Here's how the part is built. I have some questions about the finished solid (model axes, mm). A direction names the side the tool comes from. Round coordinates to 2 decimals unless told otherwise and drop trailing zeros. Loops run counter-clockwise (first coordinate to the right, second up) from the corner with the lowest first, then second, coordinate; pieces in that order, holes last. Notation, with made-up numbers: M 64,41 L 108,41 A9 ccw 108,55 Z; hole C -8,-18 d11. An arc over 180 degrees is marked long. Answer as a JSON object with one key per item and string values.
from build123d import *

# Parameters (mm, degrees)
F0_R     = 3.302
F1_DEPTH = 12.7


with BuildPart() as f1:
    # F0 (on Top) → F1 (new body)
    with BuildSketch(Plane.XY):
        with BuildLine():
            ThreePointArc((24.764251, -5.647288), (25.240562, -2.84148), (25.4, 0))
            ThreePointArc((25.4, 0), (25.399308, 0.187557), (25.39723, 0.375103))
            ThreePointArc((25.39723, 0.375103), (25.260856, 2.655023), (24.920228, 4.913475))
            ThreePointArc((24.920228, 4.913475), (24.156836, 7.849032), (23.048956, 10.672658))
            ThreePointArc((23.048956, 10.672658), (21.997045, 12.7), (20.767271, 14.624652))
            ThreePointArc((20.767271, 14.624652), (18.875879, 16.995917), (16.715308, 19.124813))
            ThreePointArc((16.715308, 19.124813), (14.929745, 20.549032), (13.023464, 21.807095))
            ThreePointArc((13.023464, 21.807095), (10.331111, 23.204055), (7.491431, 24.270115))
            ThreePointArc((7.491431, 24.270115), (5.280957, 24.844949), (3.027782, 25.218892))
            ThreePointArc((3.027782, 25.218892), (0, 25.4), (-3.027782, 25.218892))
            ThreePointArc((-3.027782, 25.218892), (-5.280957, 24.844949), (-7.491431, 24.270115))
            ThreePointArc((-7.491431, 24.270115), (-10.331111, 23.204055), (-13.023464, 21.807095))
            ThreePointArc((-13.023464, 21.807095), (-14.929745, 20.549032), (-16.715308, 19.124813))
            ThreePointArc((-16.715308, 19.124813), (-18.875879, 16.995917), (-20.767271, 14.624652))
            ThreePointArc((-20.767271, 14.624652), (-21.997045, 12.7), (-23.048956, 10.672658))
            ThreePointArc((-23.048956, 10.672658), (-24.156836, 7.849032), (-24.920228, 4.913475))
            ThreePointArc((-24.920228, 4.913475), (-25.260856, 2.655023), (-25.39723, 0.375103))
            ThreePointArc((-25.39723, 0.375103), (-25.260856, -2.655023), (-24.764251, -5.647288))
            ThreePointArc((-24.764251, -5.647288), (-24.156836, -7.849032), (-23.354093, -9.98731))
            ThreePointArc((-23.354093, -9.98731), (-21.997045, -12.7), (-20.326311, -15.231582))
            ThreePointArc((-20.326311, -15.231582), (-18.875879, -16.995917), (-17.27282, -18.622827))
            ThreePointArc((-17.27282, -18.622827), (-14.929745, -20.549032), (-12.373766, -22.182198))
            ThreePointArc((-12.373766, -22.182198), (-10.331111, -23.204055), (-8.20492, -24.038288))
            ThreePointArc((-8.20492, -24.038288), (-5.280957, -24.844949), (-2.281685, -25.29731))
            ThreePointArc((-2.281685, -25.29731), (0, -25.4), (2.281685, -25.29731))
            ThreePointArc((2.281685, -25.29731), (5.280957, -24.844949), (8.20492, -24.038288))
            ThreePointArc((8.20492, -24.038288), (10.331111, -23.204055), (12.373766, -22.182198))
            ThreePointArc((12.373766, -22.182198), (14.929745, -20.549032), (17.27282, -18.622827))
            ThreePointArc((17.27282, -18.622827), (18.875879, -16.995917), (20.326311, -15.231582))
            ThreePointArc((20.326311, -15.231582), (21.997045, -12.7), (23.354093, -9.98731))
            ThreePointArc((23.354093, -9.98731), (24.156836, -7.849032), (24.764251, -5.647288))
        make_face()
        Circle(F0_R, mode=Mode.SUBTRACT)
        with BuildLine():
            ThreePointArc((25.39723, 0.375103), (25.399308, 0.187557), (25.4, 0))
            ThreePointArc((25.4, 0), (25.240562, -2.84148), (24.764251, -5.647288))
            Line((24.764251, -5.647288), (30.631833, -3.219535))
            Line((30.631833, -3.219535), (25.39723, 0.375103))
        make_face()
        with BuildLine():
            ThreePointArc((23.048956, 10.672658), (24.156836, 7.849032), (24.920228, 4.913475))
            Line((24.920228, 4.913475), (29.293075, 9.517897))
            Line((29.293075, 9.517897), (23.048956, 10.672658))
        make_face()
        with BuildLine():
            Line((26.674069, -15.400281), (23.354093, -9.98731))
            ThreePointArc((23.354093, -9.98731), (21.997045, -12.7), (20.326311, -15.231582))
            Line((20.326311, -15.231582), (26.674069, -15.400281))
        make_face()
        with BuildLine():
            ThreePointArc((16.715308, 19.124813), (18.875879, 16.995917), (20.767271, 14.624652))
            Line((20.767271, 14.624652), (22.889278, 20.609599))
            Line((22.889278, 20.609599), (16.715308, 19.124813))
        make_face()
        with BuildLine():
            Line((18.104116, -24.918178), (17.27282, -18.622827))
            ThreePointArc((17.27282, -18.622827), (14.929745, -20.549032), (12.373766, -22.182198))
            Line((12.373766, -22.182198), (18.104116, -24.918178))
        make_face()
        with BuildLine():
            ThreePointArc((7.491431, 24.270115), (10.331111, 23.204055), (13.023464, 21.807095))
            Line((13.023464, 21.807095), (12.527717, 28.137714))
            Line((12.527717, 28.137714), (7.491431, 24.270115))
        make_face()
        with BuildLine():
            Line((6.403797, -30.127496), (8.20492, -24.038288))
            ThreePointArc((8.20492, -24.038288), (5.280957, -24.844949), (2.281685, -25.29731))
            Line((2.281685, -25.29731), (6.403797, -30.127496))
        make_face()
        with BuildLine():
            ThreePointArc((-3.027782, 25.218892), (0, 25.4), (3.027782, 25.218892))
            Line((3.027782, 25.218892), (0, 30.800562))
            Line((0, 30.800562), (-3.027782, 25.218892))
        make_face()
        with BuildLine():
            Line((-6.403797, -30.127496), (-2.281685, -25.29731))
            ThreePointArc((-2.281685, -25.29731), (-5.280957, -24.844949), (-8.20492, -24.038288))
            Line((-8.20492, -24.038288), (-6.403797, -30.127496))
        make_face()
        with BuildLine():
            ThreePointArc((-13.023464, 21.807095), (-10.331111, 23.204055), (-7.491431, 24.270115))
            Line((-7.491431, 24.270115), (-12.527717, 28.137714))
            Line((-12.527717, 28.137714), (-13.023464, 21.807095))
        make_face()
        with BuildLine():
            Line((-18.104116, -24.918178), (-12.373766, -22.182198))
            ThreePointArc((-12.373766, -22.182198), (-14.929745, -20.549032), (-17.27282, -18.622827))
            Line((-17.27282, -18.622827), (-18.104116, -24.918178))
        make_face()
        with BuildLine():
            ThreePointArc((-20.767271, 14.624652), (-18.875879, 16.995917), (-16.715308, 19.124813))
            Line((-16.715308, 19.124813), (-22.889278, 20.609599))
            Line((-22.889278, 20.609599), (-20.767271, 14.624652))
        make_face()
        with BuildLine():
            Line((-26.674069, -15.400281), (-20.326311, -15.231582))
            ThreePointArc((-20.326311, -15.231582), (-21.997045, -12.7), (-23.354093, -9.98731))
            Line((-23.354093, -9.98731), (-26.674069, -15.400281))
        make_face()
        with BuildLine():
            ThreePointArc((-24.920228, 4.913475), (-24.156836, 7.849032), (-23.048956, 10.672658))
            Line((-23.048956, 10.672658), (-29.293075, 9.517897))
            Line((-29.293075, 9.517897), (-24.920228, 4.913475))
        make_face()
        with BuildLine():
            Line((-30.631833, -3.219535), (-24.764251, -5.647288))
            ThreePointArc((-24.764251, -5.647288), (-25.260856, -2.655023), (-25.39723, 0.375103))
            Line((-25.39723, 0.375103), (-30.631833, -3.219535))
        make_face()
    extrude(amount=F1_DEPTH)


solid = f1.part
Item 1: For faces 1 (the face through (-17.683, -21.726, 6.261)), 2 (the face through (28.051, -1.447, 6.261)), 3 (the face through (-9.974, 26.177, 6.261)), which set-ups out of +Z, -Z, +X, -X, +Y, -Y let a thin tool reach every point of the face, with its end or its side?
Solution:
{"face 1": "+Z, -Z, -X", "face 2": "+Z, -Z, +X", "face 3": "+Z, -Z, +Y"}
Item 2: I want a section at A-A on x = 10. List the corners of the cut face in (y, z) for me, plus the area to 3 significant figures.
Solution:
{"outline": "M -23.35,0 L 26.2,0 L 26.2,12.7 L -23.35,12.7 Z", "area": "629 mm2"}
Item 3: We'd pull the mould along X, two halves only. Please class faces 4 (the face through (6, 1, 0)), 5 (the face through (-14.9, 20.57, 6.26)), 6 (the face through (17.694, -21.815, 6.261)), 7 (the face through (-12.77, 25.02, 6.26)): +X half, -X half, draft (parallel to the pull), parting line (faces both ways), or undercut.
Solution:
{"face 4": "draft", "face 5": "undercut", "face 6": "+X half", "face 7": "-X half"}
Item 4: If I drill on L1, parallel to Y at x = -26, z = 1.25; L2, parallel to X at y = 25.5, z = 5.5; L3, parallel to Y at x = 0.5, z = 1.5, over which ranges is the centre line in solid material (lowest first)? Write a range as from..to.
Solution:
{"L1": "y = -15.38..-14.3, -5.14..-0.04, 6.05..10.13", "L2": "x = -12.73..-9.09, -2.88..2.88, 9.09..12.73", "L3": "y = -25.4..-3.26, 3.26..29.88"}
Item 5: For P1, Ø4, axis at y = -10, z = 3, coming from the -X side; P2, Ø3, axis at x = 14.5, z = 6.5, coming from the -Y side; P3, Ø2, axis at y = 15.5, z = 3.5, coming from the -X side, each with a flat end and sliding along its axis, tell me the tip position at first contact or that it passes through.
Solution:
{"P1": "stops at x = -24.59", "P2": "stops at y = -23.91", "P3": "stops at x = -21.43"}
Item 6: I want a section at B-B on y = -8. List the corners of the cut face in (x, z) for me, plus the area to 3 significant figures.
Solution:
{"outline": "M -24.11,0 L 24.11,0 L 24.11,12.7 L -24.11,12.7 Z", "area": "612 mm2"}
